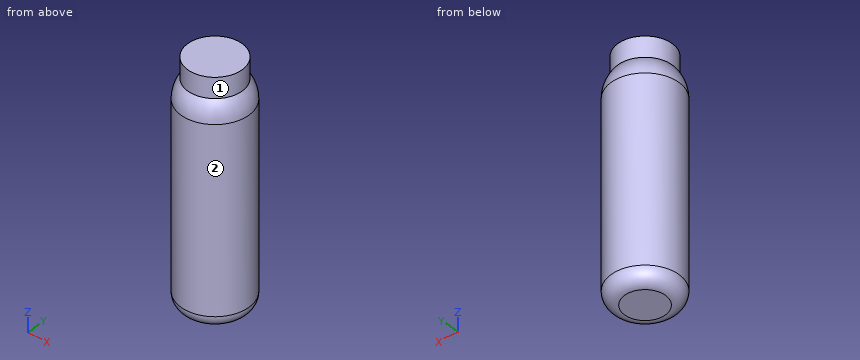
from build123d import *

# Parameters (mm, degrees)
F0_R     = 25.4
F1_DEPTH = 19.05
F2_R     = 31.75
F3_DEPTH = 203.2
F4_R     = 12.7


# Not quite as in the source:
# - a fillet or chamfer that OpenCascade refuses, or shapes differently, is made with other operations: its cross-section is extruded or revolved along the edge and cut away or added


with BuildPart() as f1:
    # F0 (on Top) → F1 (new body)
    with BuildSketch(Plane.XY):
        Circle(F0_R)
    extrude(amount=-F1_DEPTH)

    # F2 (on face) → F3 (join)
    with BuildSketch(Plane(origin=(0, 0, -19.05), x_dir=(1, 0, 0), z_dir=(0, 0, -1))):
        Circle(F2_R)
    extrude(amount=F3_DEPTH)

    # F4
    f4_edges = [f1.edges().sort_by_distance(p)[0] for p in [
        (-31.75, 0, -222.25),
    ]]
    fillet(f4_edges, radius=F4_R)

    # F5: fillet of radius 30.48 on 1 edges, made by hand

    # F5_s1 → F5_t2 (revolve, cut)
    with BuildSketch(Plane.XZ):
        with BuildLine():
            ThreePointArc((31.75, -37.6718554392), (30.1188543967, -27.8344777399), (25.4, -19.05))
            Line((25.4, -19.05), (31.75, -19.05))
            Line((31.75, -19.05), (31.75, -37.6718554392))
        make_face()
    revolve(axis=Axis((0, 0, -19.05), (0, 0, -1)), mode=Mode.SUBTRACT)


solid = f1.part
CAD build for the part. Positions are in the model's coordinates, mm. Face numbers are marked on the shaded views. A direction names the side the tool comes from. Coordinates: 2 decimals unless noted, no trailing zeros. Loops run counter-clockwise (first coordinate to the right, second up) from the corner with the lowest first, then second, coordinate; pieces in that order, holes last. Notation, with made-up numbers: (72.25, 9) - (90.25, 9) arc R4 ccw to (90.25, 13) - close; hole circle Ø9 at (-15, 18). An arc over 180 degrees is marked (long way). Write item = value, one per line. Start each with the question number.
Q1. Which spindle directions (+Z, -Z, +X, -X, +Y, -Y) get a long thin tool onto all of the face, cutting with end or side? Do the marked faces 1 and 2. Say none if no direction does.
Q2. Flat gauge pins, fed straight in: pin 1 Ø8 at (x, z) = (8, -77.5) entering from -Y; pin 2 Ø12 at (y, z) = (-15, -187.5) entering from -X; pin 3 Ø10 at (x, y) = (9, -25) entering from -Z. Where does each tip first touch, or does it go through?
Q3. Drill centre lines: L1, parallel to Z at x = 8, y = 18.5; L2, parallel to X at y = 28.5, z = -119; L3, parallel to X at y = 29, z = -197.5. Where is each one in solid material? Low to high.
Q4. Cut at A-A, the plane z = -90.5. List the corners of the cut face in (x, y), then the cut area to 3 significant figures.
Computed:
q1.face_1 = +Z
q1.face_2 = +Z, -Z
q2.pin_1 = -31.5
q2.pin_2 = -30.45
q2.pin_3 = -222
q3.L1 = -222.2 to 0
q3.L2 = -13.99 to 13.99
q3.L3 = -12.93 to 12.93
q4.outline = circle Ø63.5 at (0, 0)
q4.area = 3,170 mm²
